Part model, mm, in its own coordinate system. Face numbers are marked on the shaded views. A direction names the side the tool comes from. Coordinates: 2 decimals unless noted, no trailing zeros. Order: outer loops, then holes, each group sorted by start corner. A loop starts at its lowest first (then second) coordinate and runs counter-clockwise, first axis right, second up.
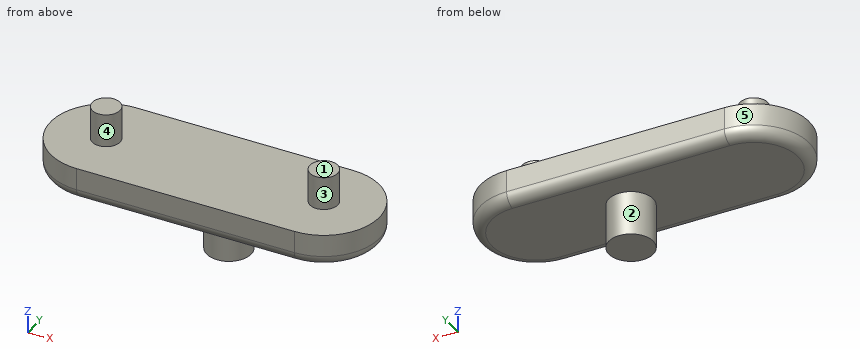
```python
from build123d import *

# Parameters (mm, degrees)
BOSS_EXTRU_1_DEPTH = 3
ESQUISSE2_R        = 1.25
BOSS_EXTRU_2_DEPTH = 3
ESQUISSE3_R        = 2
BOSS_EXTRU_3_DEPTH = 4
CONG_1_R           = 1


with BuildPart() as part:
    # Esquisse1 → Boss.-Extru.1 (new body)
    with BuildSketch(Plane.XY):
        with BuildLine():
            Line((0, -5), (-19.5, -5))
            ThreePointArc((-19.5, -5), (-24.5, 0), (-19.5, 5))
            Line((-19.5, 5), (0, 5))
            ThreePointArc((0, 5), (5, 0), (0, -5))
        make_face()
    extrude(amount=BOSS_EXTRU_1_DEPTH)

    # Esquisse2 → Boss.-Extru.2 (add)
    with BuildSketch(Plane.XY.offset(3)):
        with Locations((-19.5, 0)):
            Circle(ESQUISSE2_R)
        Circle(ESQUISSE2_R)
    extrude(amount=BOSS_EXTRU_2_DEPTH)

    # Esquisse3 → Boss.-Extru.3 (add)
    with BuildSketch(Plane(origin=(0, 0, 0), x_dir=(-1, 0, 0), z_dir=(0, 0, -1))):
        with Locations(Location((8.5, 0, 0), (0, 0, 180))):
            Circle(ESQUISSE3_R)
    extrude(amount=BOSS_EXTRU_3_DEPTH)

    # Congé1
    cong_1_edges = [part.edges().sort_by_distance(p)[0] for p in [
        (-9.75, -5, 0),
        (-24.5, 0, 0),
        (-9.75, 5, 0),
        (5, 0, 0),
    ]]
    fillet(cong_1_edges, radius=CONG_1_R)


solid = part.part
```
(1) Slice it at D-D, the plane z = -1.5. Give the cut face in (x, y).
(2) Slice it at C-C, the plane z = 4.25. Give the cut face in (x, y).
(3) Pull direction X, two halves, no side cores. Call the marked faces 1, 2 and 3: +X half, -X half, draft (parallel to the pull), parting line (faces both ways), or undercut.
(4) Slice it at B-B, the plane y = 0. Give the cut face in (x, z).
(5) Slice it at A-A, the plane x = -8.5. Give the cut face in (y, z).
(6) Probe line 1 (Z direction, x = -1.5, y = 1.5); line 2 (Y direction, x = 3, z = 1.5); line 3 (X direction, y = -2, z = 2.5). List the from-to ranges inside material, lowest first.
(7) Tool access for the marked faces 4 and 5: list every direction of +Z, -Z, +X, -X, +Y, -Y with a clear straight run to the whole face (end or side of a thin tool).
(8) Drop flat-ended pins along their axis: pin 1 (6 mm diameter, centred on x = -8.5, y = 2.5, fed in from +Z); pin 2 (3 mm diameter, centred on y = 3, z = -2.5, fed in from +X). Give the stop position or say it passes through.
Here are the results:
1. outline: circle Ø4 at (-8.5, 0)
2. outline: circle Ø2.5 at (-19.5, 0); circle Ø2.5 at (0, 0)
3. face 1: draft
3. face 2: parting line
3. face 3: undercut
4. outline: (-24.5, 1) arc R1 ccw to (-23.5, 0) - (-10.5, 0) - (-10.5, -4) - (-6.5, -4) - (-6.5, 0) - (4, 0) arc R1 ccw to (5, 1) - (5, 3) - (1.25, 3) - (1.25, 6) - (-1.25, 6) - (-1.25, 3) - (-18.25, 3) - (-18.25, 6) - (-20.75, 6) - (-20.75, 3) - (-24.5, 3) - close
5. outline: (-5, 1) arc R1 ccw to (-4, 0) - (-2, 0) - (-2, -4) - (2, -4) - (2, 0) - (4, 0) arc R1 ccw to (5, 1) - (5, 3) - (-5, 3) - close
6. line 1: z = 0 to 3
6. line 2: y = -4 to 4
6. line 3: x = -24.08 to 4.58
7. face 4: +Z
7. face 5: +Z, -Z, -X
8. pin 1: stops at z = 3
8. pin 2: stops at x = -7.18
